Model file for the job. Use its own axes, mm. Face numbers are marked on the shaded views. A direction names the side the tool comes from. Give positions to 0.01 mm unless a question says otherwise; leave off trailing zeros. Loops run counter-clockwise (first coordinate to the right, second up) from the corner with the lowest first, then second, coordinate; pieces in that order, holes last. Notation, with made-up numbers: M 6,-1 L 38,-1 A27 cw 38,21 Z; hole C 54,49.25 d1. An arc over 180 degrees is marked long. Answer in a Markdown table with one row per item.
Autodesk Fusion 360 part; units mm, degrees
sketch "Sketch1" plane through (0, 0, 0) normal (0, 0, 1) x (1, 0, 0)
  line L0 (-65, 30) -> (65, 30)
  line L1 (65, 30) -> (65, -70)
  line L2 (65, -70) -> (-65, -70)
  line L3 (-65, -70) -> (-65, 30)
  dimension "d1" = 130
  dimension "d2" = 100
extrude "Extrude1" add sketch "Sketch1" along normal blind 25
sketch "Sketch3" plane through (-65, 0, 0) normal (-1, 0, 0) x (0, -1, 0)
  line L0 (-30, 0) -> (70, 0)
  line L1 (70, 0) -> (70, 25)
  line L2 (70, 25) -> (-30, 25)
  line L3 (-30, 25) -> (-30, 0)
  circle A0 centre (-20.2556, 10) radius 4
  circle A1 centre (59.7444, 10) radius 4
  dimension "d6" = 8
  dimension "d7" = 10
  dimension "d8" = 80
extrude "Extrude2" cut sketch "Sketch3" against normal blind 10 contours A0 | A1
sketch "Sketch4" plane through (0, -70, 0) normal (0, -1, 0) x (1, 0, 0)
  line L0 (-65, 0) -> (65, 0)
  line L1 (65, 0) -> (65, 25)
  line L2 (65, 25) -> (-65, 25)
  line L3 (-65, 25) -> (-65, 0)
  line L4 (-55, 0) -> (-5, 0)
  line L5 (-5, 0) -> (-5, 20)
  line L6 (-5, 20) -> (-55, 20)
  line L7 (-55, 20) -> (-55, 0)
  dimension "d11" = 10
  dimension "d12" = 20
  dimension "d15" = 50
extrude "Extrude3" cut sketch "Sketch4" against normal blind 20 contours L0 L4 L5 L6 L7
sketch "Sketch5" plane through (0, 30, 0) normal (0, 1, 0) x (-1, 0, 0)
  line L0 (-65, 0) -> (65, 0)
  line L1 (65, 0) -> (65, 25)
  line L2 (65, 25) -> (-65, 25)
  line L3 (-65, 25) -> (-65, 0)
  line L4 (5, 20) -> (55, 20)
  line L5 (55, 20) -> (55, 0)
  line L6 (55, 0) -> (5, 0)
  line L7 (5, 0) -> (5, 20)
  dimension "d16" = 50
  dimension "d17" = 20
  dimension "d19" = 10
extrude "Extrude4" cut sketch "Sketch5" against normal blind 20 contours L0 L4 L5 L6 L7
sketch "Sketch6" plane through (0, -70, 0) normal (0, -1, 0) x (1, 0, 0)
  line L0 (-55, 0) -> (-55, 20)
  line L1 (-55, 20) -> (-5, 20)
  line L2 (-5, 20) -> (-5, 0)
  line L3 (-5, 0) -> (65, 0)
  line L4 (65, 0) -> (65, 25)
  line L5 (65, 25) -> (-65, 25)
  line L6 (-65, 25) -> (-65, 0)
  line L7 (-65, 0) -> (-55, 0)
  line L8 (9.1818, 0) -> (65, 20.3162)
  dimension "d22" = 20
extrude "Extrude5" cut sketch "Sketch6" against normal through all contours L3 L4 L8
sketch "Sketch7" plane through (0, -70, 0) normal (0, -1, 0) x (1, 0, 0)
  line L0 (9.1818, 0) -> (65, 20.3162)
  line L1 (65, 20.3162) -> (65, 25)
  line L2 (65, 25) -> (-65, 25)
  line L3 (-65, 25) -> (-65, 0)
  line L4 (-65, 0) -> (-55, 0)
  line L5 (-55, 0) -> (-55, 20)
  line L6 (-55, 20) -> (-5, 20)
  line L7 (-5, 20) -> (-5, 0)
  line L8 (-5, 0) -> (9.1818, 0)
  line L9 (0, 20) -> (0, 5)
  line L10 (0, 5) -> (9.1818, 5)
  line L11 (9.1818, 5) -> (0, 20)
  line L12 (4.966, 20) -> (55.36, 20)
  line L13 (55.36, 20) -> (14.1478, 5)
  line L14 (14.1478, 5) -> (4.966, 20)
  dimension "d24" = 5
  dimension "d25" = 5
  dimension "d27" = 3
extrude "Extrude6" cut sketch "Sketch7" against normal through all contours L9 L10 L11 | L12 L13 L14
sketch "Sketch8" plane through (0, -50, 0) normal (0, -1, 0) x (1, 0, 0)
  line L0 (-55, 20) -> (-55, 0)
  line L1 (-55, 0) -> (-5, 0)
  line L2 (-5, 0) -> (-5, 20)
  line L3 (-5, 20) -> (-55, 20)
  line L4 (-45, 20) -> (-30, 5)
  line L5 (-30, 5) -> (-15, 20)
  line L6 (-45, 20) -> (-15, 20)
  dimension "d29" = 45
  dimension "d30" = 45
  dimension "d31" = 5
extrude "Extrude7" cut sketch "Sketch8" against normal through all contours L3 L4 L5 L6
sketch "Sketch9" plane through (0, -50, 0) normal (0, -1, 0) x (1, 0, 0)
  line L0 (-30, 5) -> (-45, 20)
  line L1 (-45, 20) -> (-55, 20)
  line L2 (-55, 20) -> (-55, 0)
  line L3 (-55, 0) -> (-5, 0)
  line L4 (-5, 0) -> (-5, 20)
  line L5 (-5, 20) -> (-15, 20)
  line L6 (-15, 20) -> (-30, 5)
  line L7 (-50, 15) -> (-50, 5)
  line L8 (-50, 5) -> (-37.0711, 5)
  line L9 (-37.0711, 5) -> (-47.0711, 15)
  line L10 (-47.0711, 15) -> (-50, 15)
  line L11 (-30, 13.9289) -> (-30, -2.0711)
  line L12 (-12.9289, 15) -> (-10, 15)
  line L13 (-10, 15) -> (-10, 5)
  line L14 (-10, 5) -> (-22.9289, 5)
  line L15 (-22.9289, 5) -> (-12.9289, 15)
  dimension "d33" = 5
  dimension "d34" = 5
  dimension "d35" = 5
  dimension "d36" = 5
extrude "Extrude8" cut sketch "Sketch9" against normal through all contours L7 L8 L9 L10 | L12 L13 L14 L15
sketch "Sketch10" plane through (0, 0, 25) normal (0, 0, 1) x (-1, 0, 0)
  line L0 (65, 70) -> (-65, 70)
  line L1 (-65, 70) -> (-65, -30)
  line L2 (-65, -30) -> (65, -30)
  line L3 (65, -30) -> (65, 70)
  circle A0 centre (0, 20) radius 7.5
  point P0 (0, -30)
  point P1 (65, 20)
  dimension "d38" = 15
extrude "Extrude9" add sketch "Sketch10" along normal blind 10 contours A0
fillet "Fillet1" radius 2 1 edges at (6.9925, -17.2879, 35)
fillet "Fillet1" radius 2 4 edges at (65, -20, 20.3162) (14.1478, -20, 5) (55.36, -20, 20) (4.966, -20, 20)
fillet "Fillet1" radius 0.5 3 edges at (9.1818, -20, 5) (0, -20, 5) (0, -20, 20)
fillet "Fillet1" radius 0.5 4 edges at (-10, -20, 5) (-10, -20, 15) (-12.9289, -20, 15) (-22.9289, -20, 5)
fillet "Fillet1" radius 0.5 4 edges at (-37.0711, -20, 5) (-50, -20, 5) (-50, -20, 15) (-47.0711, -20, 15)
fillet "Fillet1" radius 2 1 edges at (-30, -20, 5)
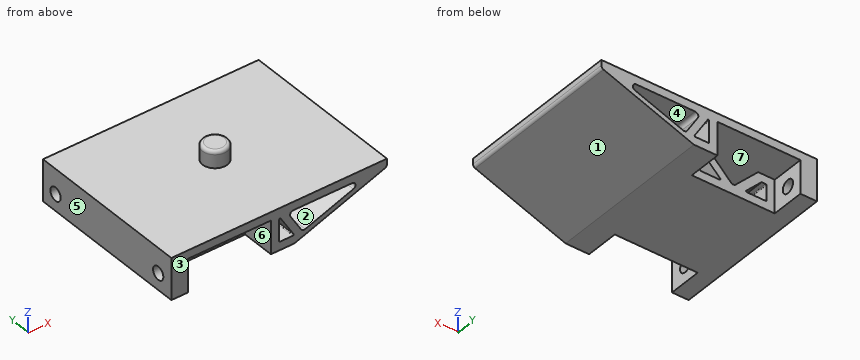
Q1. Probe probe 1 along Z at (x, y) = (-25.5, 14.5); probe 2 along Z at (x, y) = (27.5, -20); probe 3 along Z at (x, y) = (3.5, 2.5). List the from-to ranges inside material, lowest first.
Reported:
| item | result |
|---|---|
| probe 1 | 20 to 25 |
| probe 2 | 6.67 to 9.86, 20 to 25 |
| probe 3 | 0 to 5, 14.28 to 25 |
Q2. Saw through at C-C (x = -53). Give the cut face in (y, z).
Reported:
| item | result |
|---|---|
| outline | M -70,20 L -50,20 L -50,0 L 10,0 L 10,20 L 30,20 L 30,25 L -70,25 Z |
Q3. 3-axis set-ups, long thin cutter, end or side, ignore diameter. For the marked faces 4, 5, 6 and 7: which of +Z, -Z, +X, -X, +Y, -Y reach the whole face in a straight line?
Reported:
| item | result |
|---|---|
| face 4 | +Y, -Y |
| face 5 | +Z, -Z, -X, +Y, -Y |
| face 6 | -Z, -Y |
| face 7 | none |
Q4. Saw through at B-B (x = 34.5). Give the cut face in (y, z).
Reported:
| item | result |
|---|---|
| outline | M -70,9.22 L 30,9.22 L 30,12.41 L -70,12.41 Z; M -70,20 L 30,20 L 30,25 L -70,25 Z |
Q5. Mould opens along X. For the marked faces 1, 2 and 3 say: released by +X, released by -X, zero draft, split by the parting line, or undercut.
Reported:
| item | result |
|---|---|
| face 1 | released by +X |
| face 2 | undercut |
| face 3 | zero draft |
Q6. Drop flat-ended pins along their axis: pin 1 (16 mm diameter, centred on x = -36, z = 11, fed in from -Y); pin 2 (1 mm diameter, centred on x = -12, z = 7, fed in from +Y); pin 3 (16 mm diameter, centred on y = 20.5, z = 13.5, fed in from +X); pin 4 (4 mm diameter, centred on x = 6.5, y = -10.5, fed in from +Z). Give the stop position or say it passes through.
Reported:
| item | result |
|---|---|
| pin 1 | y = -50 |
| pin 2 | through |
| pin 3 | x = 64.99 |
| pin 4 | z = 25 |
Q7. Saw through at D-D (y = -3). Give the number of separate pieces and of enclosed holes in the cut face, and give its area (3 significant figures).
Reported:
| item | result |
|---|---|
| separate pieces | 1 |
| enclosed holes | 5 |
| area | 1,880 mm² |
Q8. Saw through at A-A (y = 19). Give the cut face in (x, z), and give its area (3 significant figures).
Reported:
| item | result |
|---|---|
| outline | M -65,0 L -55,0 L -55,6.2 L -65,6.2 Z; M -65,13.8 L -55,13.8 L -55,20 L -5,20 L -5,0 L 9.18,0 L 63.68,19.84 A2 ccw 65,21.72 L 65,25 L -65,25 Z; hole M 0,5.5 A0.5 ccw 0.5,5 L 8.29,5 A0.5 ccw 8.72,5.76 L 0.93,18.49 A0.5 ccw 0,18.23 Z; hole M 6.83,16.96 L 13.29,6.39 A2 ccw 15.68,5.56 L 44.7,16.12 A2 ccw 44.02,20 L 8.54,20 A2 ccw Z |
| area | 1,180 mm² |
